Geometry: final body of the model. Coordinates: model frame, mm. Give positions to 0.01 mm unless a question says otherwise; leave off trailing zeros. Write each loop counter-clockwise with the first axis right and the second up, starting at its lowest first coordinate (ties: lowest second). Pieces come first, ordered by that corner, then holes. Notation, with made-up numbers: M 31.25,-5.5 L 55.25,-5.5 A14 ccw 55.25,17.5 Z; hole C 39.25,2.25 d8. An arc over 180 degrees is marked long. Use one line per item in the form item = value. Start each with the question number.
Item 1: Material intervals for line 1 along Z through (x, y) = (7, 13); line 2 along Y through (x, z) = (-39.5, -12.6); line 3 along Y through (x, z) = (-33, -12.6), sorted ascending. Write a range as from..to.
Item 2: Section query D-D on z = -11.3. Return loops of the section in (x, y), then the cut area to 3 significant figures.
Item 3: Section query B-B on x = 0.5. Return loops of the section in (y, z), then the cut area to 3 significant figures.
Item 4: Contact query for flat-ended pins moving along their axis: P1, Ø3.5, axis at x = -49.5, y = 2.5, coming from the +Z side; P2, Ø2.5, axis at x = 10, y = 0.5, coming from the +Z side; P3, Ø1.1, axis at y = 18.5, z = -12.5, coming from the +X side; P4, Ø6.5, axis at x = 6, y = 29.5, coming from the -Z side. Output: stop coordinate, or through.
Item 5: Section query A-A on y = 7. Return loops of the section in (x, z).
Item 6: Section query C-C on y = 13.5. Return loops of the section in (x, z).
from build123d import *

# Parameters (mm, degrees)
PAD027_DEPTH    = 1
SKETCH043_W     = 3.05
SKETCH043_H     = 8.1
SKETCH043_W_2   = 8.1
SKETCH043_H_2   = 3.05
POCKET016_DEPTH = 0.5
POCKET017_DEPTH = 0.25
POCKET018_DEPTH = 0.25
CHAMFER007_SIZE = 0.25
SKETCH046_W     = 8
SKETCH046_H     = 3
PAD028_DEPTH    = 0.5
SKETCH047_R     = 1.55
SKETCH047_R_2   = 1.75
PAD029_DEPTH    = 3


with BuildPart() as part:
    # Sketch042 (on Face1 of Binder013) → Pad027 (new body)
    with BuildSketch(Plane(origin=(0, 0, -13), x_dir=(1, 0, 0), z_dir=(0, 0, -1))):
        Polygon((13, -5.333333), (13, -23.333333), (2.352991501, -33.980341499), (2.352991501, -47.019624501), (-41.313708499, -47.019624501), (-61, -35.6537388036), (-61, -3.6537388036), (-35, -3.6537388036), (-21.4834043405, 4.1500713405), (3.5165956595, 4.1500713405), align=None)
    extrude(amount=-PAD027_DEPTH)

    # Sketch043 (on Face11 of Pad027) → Pocket016 (cut)
    with BuildSketch(Plane(origin=(0, 0, -13), x_dir=(1, 0, 0), z_dir=(0, 0, -1))):
        with Locations((11.475, -14.333333)):
            Rectangle(SKETCH043_W, SKETCH043_H)
        with Locations((0.827991501, -38.979624501)):
            Rectangle(SKETCH043_W, SKETCH043_H)
        with Locations((-5.322008499, -45.494624501)):
            Rectangle(SKETCH043_W_2, SKETCH043_H_2)
        with Locations((-27.713708499, -45.494624501)):
            Rectangle(SKETCH043_W_2, SKETCH043_H_2)
        Polygon((-54.5481107418, -39.3787388036), (-47.5333049711, -43.4287388036), (-46.0083049711, -40.787361322), (-53.0231107418, -36.737361322), align=None)
        Polygon((10.5200748237, -25.8132581763), (4.7925098961, -31.5408231039), (2.6358342135, -29.3841474213), (8.3633991411, -23.6565824937), align=None)
    extrude(amount=-POCKET016_DEPTH, mode=Mode.SUBTRACT)

    # Sketch044 (on Face7 of Pocket016) → Pocket017 (cut)
    with BuildSketch(Plane.XY.offset(-12)):
        Polygon((13, 5.333333), (3.5165956595, -4.1500713405), (-21.4834043405, -4.1500713405), (-35, 3.6537388036), (-61, 3.6537388036), (-61, 4.1537388036), (-34.8660254038, 4.1537388036), (-21.3494297442, -3.6500713405), (3.3094888783, -3.6500713405), (13, 6.0404397812), align=None)
    extrude(amount=-POCKET017_DEPTH, mode=Mode.SUBTRACT)

    # Sketch045 (on Face7 of Pocket017) → Pocket018 (cut)
    with BuildSketch(Plane.XY.offset(-12)):
        Polygon((2.352991501, 33.980341499), (-20.3541152802, 33.980341499), (-34.8660254038, 19.4684313754), (-34.8660254038, 4.1537388036), (-34.3660254038, 3.8650636689), (-34.3660254038, 19.2613245942), (-20.147008499, 33.480341499), (2.852991501, 33.480341499), align=None)
    extrude(amount=-POCKET018_DEPTH, mode=Mode.SUBTRACT)

    # Chamfer007
    chamfer007_edges = [part.edges().sort_by_distance(p)[0] for p in [
        (-61, 19.903739, -12),
    ]]
    chamfer(chamfer007_edges, length=CHAMFER007_SIZE)

    # Sketch046 (on Face4 of Chamfer007) → Pad028 (join)
    with BuildSketch(Plane(origin=(0, 0, -13), x_dir=(1, 0, 0), z_dir=(0, 0, -1))):
        with Locations((-51, -2.1537388036)):
            Rectangle(SKETCH046_W, SKETCH046_H)
        with Locations((-8.9834043405, 5.6500713405)):
            Rectangle(SKETCH046_W, SKETCH046_H)
        Polygon((-24.7809002358, 2.2462611973), (-31.7091034658, -1.7537388033), (-33.209103466, 0.8443374079), (-26.2809002361, 4.8443374085), align=None)
        Polygon((11.0826382182, -3.4159712182), (5.4257839687, 2.2408830313), (7.5471043123, 4.3622033748), (13.2039585618, -1.2946508747), align=None)
    extrude(amount=-PAD028_DEPTH)

    # Sketch047 (on Face63 of Pad028) → Pad029 (join)
    with BuildSketch(Plane.XY.offset(-12)):
        with Locations((0.5, 27.793333)):
            Circle(SKETCH047_R)
        with Locations((1, 20.993333)):
            Circle(SKETCH047_R_2)
    extrude(amount=PAD029_DEPTH)


solid = part.part
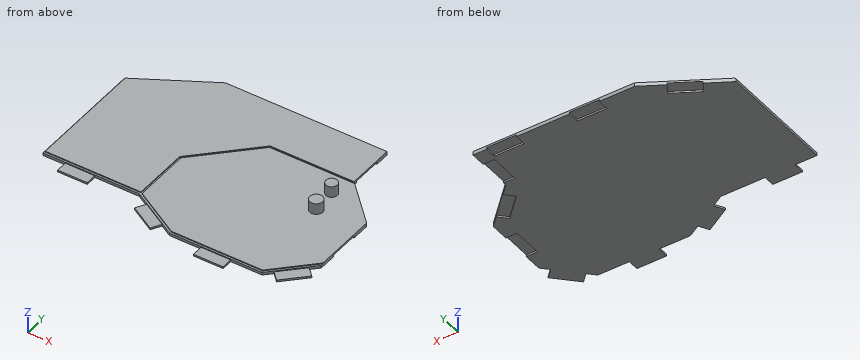
Answer sheet:
q1.line_1 = -13..-12
q1.line_2 = 3.65..47.02
q1.line_3 = -0.97..-0.48, 2.5..47.02
q2.outline = C 0.5,27.79 d3.1; C 1,20.99 d3.5
q2.area = 17.2 mm2
q3.outline = M -4.15,-13 L 34.93,-13 L 34.93,-12.5 L 43.03,-12.5 L 43.03,-13 L 47.02,-13 L 47.02,-12 L 33.98,-12 L 33.98,-12.25 L 33.48,-12.25 L 33.48,-12 L 29.34,-12 L 29.34,-9 L 26.24,-9 L 26.24,-12 L 22.67,-12 L 22.67,-9 L 19.32,-9 L 19.32,-12 L -3.65,-12 L -3.65,-12.25 L -4.15,-12.25 Z
q3.area = 66.2 mm2
q4.P1 = -12
q4.P2 = -12.5
q4.P3 = 13
q4.P4 = -13
q5.outline = M -61,-13 L 13,-13 L 13,-12 L -34.37,-12 L -34.37,-12.25 L -34.87,-12.25 L -34.87,-12 L -60.75,-12 L -61,-12.25 Z
q6.outline = M -61,-13 L 9.95,-13 L 9.95,-12.5 L 13,-12.5 L 13,-12 L -34.37,-12 L -34.37,-12.25 L -34.87,-12.25 L -34.87,-12 L -60.75,-12 L -61,-12.25 Z
